from build123d import *

# Parameters (mm, degrees)
F0_R      = 75.3383577212
F1_DEPTH  = 76.2
F2_R      = 37.9498660495
F3_DEPTH  = 127
F5_R      = 18.6285804239
F6_DEPTH  = 76.2
F4_R      = 37.9498660495
F7_DEPTH  = 76.2
F8_DEPTH  = 50.8
F9_R      = 16.6862695849
F10_DEPTH = 76.2


with BuildPart() as f1:
    # F0 (on Front) → F1 (new body)
    with BuildSketch(Plane.XZ):
        Circle(F0_R)
    extrude(amount=F1_DEPTH)

    # F2 (on Front) → F3 (join)
    with BuildSketch(Plane.XZ):
        with Locations((3.9345594123, 0)):
            Circle(F2_R)
    extrude(amount=F3_DEPTH)

    # F5 (on face) → F6 (cut)
    with BuildSketch(Plane.XZ.offset(127)):
        Circle(F5_R)
    extrude(amount=-F6_DEPTH, mode=Mode.SUBTRACT)

    # F4 (on face) → F7 (join)
    with BuildSketch(Plane.XZ.offset(127)):
        with Locations((3.9345594123, 0)):
            Circle(F4_R)
    extrude(amount=F7_DEPTH)

    # F8 (cut): a face of the model
    f8_faces = [f1.faces().sort_by_distance(p)[0] for p in [
        (3.9345594123, -203.2, 0),
    ]]
    extrude(f8_faces, amount=-F8_DEPTH, mode=Mode.SUBTRACT)

    # F9 (on face) → F10 (cut)
    with BuildSketch(Plane.XZ.offset(152.4)):
        with Locations((6.8308734335, -2.1039112471)):
            Circle(F9_R)
    extrude(amount=-F10_DEPTH, mode=Mode.SUBTRACT)


solid = f1.part
For this review, take the finished solid that the model builds, in its own axes (mm). A direction names the side the tool comes from. Give positions to 0.01 mm unless a question says otherwise; leave off trailing zeros. Loops run counter-clockwise (first coordinate to the right, second up) from the corner with the lowest first, then second, coordinate; pieces in that order, holes last.
Item 1: Tool access review of faces 4 (the cylindrical face through (22.245, -123.3, -8.495)), 5 (the flat face through (-13, -152.4, 1)), 6 (the flat face through (0, -50.8, 0)): name each direction out of +Z, -Z, +X, -X, +Y, -Y from which nothing blocks a thin tool from reaching the whole face with its end or side.
Item 2: Take a section at A-A, the plane z = -12.5. State the section outline as (x, y) points, and give its area (3 significant figures).
Item 3: Take a section at B-B, the plane y = -57.5. State the section outline as (x, z) points, and give its area (3 significant figures).
Item 4: Take a section at C-C, the plane x = 0. State the section outline as (y, z) points, and give its area (3 significant figures).
Item 5: Insertion check: pin 1 (1.5 mm diameter, centred on y = -31, z = -56.5, fed in from -X); pin 2 (4 mm diameter, centred on y = -122, z = -6.5, fed in from -X); pin 3 (12 mm diameter, centred on y = -66, z = -36.5, fed in from -X). Each pin has a flat end and moves straight along its axis. Give the tip position at first contact, or say it passes through.
Item 6: Take a section at D-D, the plane y = -18. State the section outline as (x, z) points, and give its area (3 significant figures).
Item 7: Draft analysis for pull direction Z (two halves, no side actions). For faces 1 (the cylindrical face through (-59.79, -37.57, -45.84)), 2 (the flat face through (-1, 0, 1)), 3 (the flat face through (-10, -127, 1)), state which applies: +Z half, -Z half, draft (parallel to the pull), parting line (faces both ways), or undercut.
Item 8: For line 1 along Y through (x, z) = (4, 15.5); line 2 along Z through (x, y) = (0, -67); line 3 along Z through (x, y) = (2, -45.5), list the stretches that pass through material, from the lowest coordinate up.
Calculated:
1. face 4: -Y
1. face 5: +Z, -Z, +X, -X, -Y
1. face 6: none
2. outline: (-74.29, -76.2) - (-31.9, -76.2) - (-31.9, -152.4) - (-6.22, -152.4) - (-6.22, -127) - (-13.81, -127) - (-13.81, -50.8) - (13.81, -50.8) - (13.81, -76.2) - (19.88, -76.2) - (19.88, -152.4) - (39.77, -152.4) - (39.77, -76.2) - (74.29, -76.2) - (74.29, 0) - (-74.29, 0) - close
2. area: 13,700 mm2
3. outline: circle Ø150.68 at (0, 0); hole circle Ø37.26 at (0, 0)
3. area: 16,700 mm2
4. outline: (-152.4, -37.75) - (-76.2, -37.75) - (-76.2, -75.34) - (0, -75.34) - (0, 75.34) - (-76.2, 75.34) - (-76.2, 37.75) - (-152.4, 37.75) - (-152.4, 13.12) - (-127, 13.12) - (-127, 18.63) - (-50.8, 18.63) - (-50.8, -18.63) - (-127, -18.63) - (-127, -17.33) - (-152.4, -17.33) - close
4. area: 13,600 mm2
5. pin 1: stops at x = -50.67
5. pin 2: stops at x = -33.75
5. pin 3: stops at x = -68.89
6. outline: circle Ø150.68 at (0, 0)
6. area: 17,800 mm2
7. face 1: parting line
7. face 2: draft
7. face 3: undercut
8. line 1: y = -152.4 to -127, -50.8 to 0
8. line 2: z = -75.34 to -18.63, 18.63 to 75.34
8. line 3: z = -75.31 to 75.31
